from build123d import *

# Parameters (mm, degrees)
SURFACE_SKETCH_W         = 22.5
SURFACE_SKETCH_H         = 30
BODY_DEPTH               = 4.5
SKETCH_19_W              = 22.5
SKETCH_19_H              = 24
EXTRUDE_4_DEPTH          = 3
FILLET_6_R               = 1.5
MAGNET_CUTOUT_SKETCH_W   = 2.2
MAGNET_CUTOUT_SKETCH_H   = 6.2
MAGNET_CUTOUT_DEPTH      = 2.6
BORDER_DEPTH             = 0.5
CHAMPFER_DEPTH           = 22.5
FILLET_7_R               = 1.5
FILLET_8_R               = 0.5
CUT_EXTRUDE_1_DEPTH      = 23.5
CUT_EXTRUDE_2_DEPTH      = 1
CUT_EXTRUDE_2_DEPTH_BACK = 55


with BuildPart() as part:
    # surface_sketch → body (new body)
    with BuildSketch(Plane(origin=(0, 0, 0), x_dir=(1, 0, 0), z_dir=(0, 1, 0))):
        with Locations((-1.15, 0)):
            Rectangle(SURFACE_SKETCH_W, SURFACE_SKETCH_H)
    extrude(amount=-BODY_DEPTH)

    # Эскиз19 → Бобышка-Вытянуть4 (add)
    with BuildSketch(Plane(origin=(0, -4.5, 0), x_dir=(1, 0, 0), z_dir=(0, 1, 0))):
        with Locations((-1.15, -27)):
            Rectangle(SKETCH_19_W, SKETCH_19_H)
    extrude(amount=EXTRUDE_4_DEPTH)

    # Скругление6
    fillet_6_edges = [part.edges().sort_by_distance(p)[0] for p in [
        (-12.4, -3, 39),
        (10.1, -3, 39),
        (10.1, -2.25, -15),
        (-12.4, -2.25, -15),
    ]]
    fillet(fillet_6_edges, radius=FILLET_6_R)

    # magnet_cutout_sketch → magnet_cutout (cut)
    with BuildSketch(Plane.XZ.offset(4.5)):
        with Locations((9, 7.1)):
            Rectangle(MAGNET_CUTOUT_SKETCH_W, MAGNET_CUTOUT_SKETCH_H)
    magnet_cutout = extrude(amount=-MAGNET_CUTOUT_DEPTH, mode=Mode.SUBTRACT)

    # magnet_cutout_mirror: magnet_cutout across plane
    add(magnet_cutout.mirror(Plane(origin=(-1.15, 0, 0), x_dir=(0, 0, 1), z_dir=(1, 0, 0))), mode=Mode.SUBTRACT)

    # border_sketch → border (add)
    with BuildSketch(Plane(origin=(0, 0, 0), x_dir=(1, 0, 0), z_dir=(0, 1, 0))):
        with BuildLine():
            Line((-12.4, -15), (-12.4, 13.5))
            ThreePointArc((-12.4, 13.5), (-11.960660172, 14.560660172), (-10.9, 15))
            Line((-10.9, 15), (8.6, 15))
            ThreePointArc((8.6, 15), (9.660660172, 14.560660172), (10.1, 13.5))
            Line((10.1, 13.5), (10.1, -15))
            Line((10.1, -15), (9.1, -15))
            Line((9.1, -15), (9.1, 13.5))
            ThreePointArc((9.1, 13.5), (8.953553391, 13.853553391), (8.6, 14))
            Line((8.6, 14), (-10.9, 14))
            ThreePointArc((-10.9, 14), (-11.253553391, 13.853553391), (-11.4, 13.5))
            Line((-11.4, 13.5), (-11.4, -15))
            Line((-11.4, -15), (-12.4, -15))
        make_face()
    extrude(amount=BORDER_DEPTH)

    # Эскиз21 → champfer (add)
    with BuildSketch(Plane.ZY.offset(12.4)):
        Polygon((15, 0.5), (17, -1.5), (15, -1.5), (14, -1.5), (14, 0.5), align=None)
    extrude(amount=-CHAMPFER_DEPTH)

    # Скругление7
    fillet_7_edges = [part.edges().sort_by_distance(p)[0] for p in [
        (-12.4, -0.5, 16),
        (10.1, -0.5, 16),
    ]]
    fillet(fillet_7_edges, radius=FILLET_7_R)

    # Скругление8
    fillet_8_edges = [part.edges().sort_by_distance(p)[0] for p in [
        (9.1, 0.25, 14),
        (-11.4, 0.25, 14),
    ]]
    fillet(fillet_8_edges, radius=FILLET_8_R)

    # Эскиз22 → Вырез-Вытянуть1 (cut, through all)
    with BuildSketch(Plane.ZY.offset(12.4)):
        with BuildLine():
            Line((12.878679656, 0.5), (14.378679656, 0.5))
            ThreePointArc((14.378679656, 0.5), (14.952704805, 0.385819299), (15.439339828, 0.060660172))
            Line((15.439339828, 0.060660172), (17, -1.5))
            Line((17, -1.5), (17.923275361, -1.5))
            Line((17.923275361, -1.5), (15.181180077, 1.242095285))
            Line((15.181180077, 1.242095285), (12.878679656, 1.122407091))
            Line((12.878679656, 1.122407091), (12.878679656, 0.5))
        make_face()
    extrude(amount=-CUT_EXTRUDE_1_DEPTH, mode=Mode.SUBTRACT)

    # Эскиз23 → Вырез-Вытянуть2 (cut, two sides)
    with BuildSketch(Plane(origin=(0, 0, -15), x_dir=(-1, 0, 0), z_dir=(0, 0, -1))) as cut_extrude_2_sk:
        Polygon((1.15, -4.5), (-0.85, -4.5), (1.15, -2.5), (3.15, -4.5), align=None)
    extrude(amount=CUT_EXTRUDE_2_DEPTH, mode=Mode.SUBTRACT)
    extrude(cut_extrude_2_sk.sketch, amount=-CUT_EXTRUDE_2_DEPTH_BACK, mode=Mode.SUBTRACT)


solid = part.part
Can you work these out from the model? Positions are in its coordinate system, mm. A direction names the side the tool comes from. Give positions to 0.01 mm unless a question says otherwise; leave off trailing zeros. Loops run counter-clockwise (first coordinate to the right, second up) from the corner with the lowest first, then second, coordinate; pieces in that order, holes last. Notation, with made-up numbers: (20.5, -30) -> (35.5, -30) arc R28 ccw to (35.5, 2) -> close; hole circle Ø10 at (69, -13.5). An arc over 180 degrees is marked (long way). Use one line per item in the form item = value.
1) I need wall thicknesses on line 1 along Z through (x, y) = (0.75, 0.05); line 2 along X through (y, z) = (0.2, 11); line 3 along Z through (x, y) = (8.5, -3.15). Which ranges of each line are inside material? Lowest first, please.
Answers:
line_1 = -15 to -14, 14 to 15.45
line_2 = -12.4 to -11.4, 9.1 to 10.1
line_3 = -15 to 4, 10.2 to 39
2) Will these pins go through, and if not, where does the flat tip stop? pin 1 (2 mm diameter, centred on y = -3, z = 8.5, fed in from -X); pin 2 (1.1 mm diameter, centred on x = -11.5, z = 8.5, fed in from -Y); pin 3 (7 mm diameter, centred on x = -6, z = 27.5, fed in from +Y).
Answers:
pin_1 = -10.2
pin_2 = -1.9
pin_3 = -1.5
3) If we section it at B-B (z = 12): Please give me the cut outline in (x, y), plus the area to 4 significant figures.
Answers:
outline = (-12.4, -4.5) -> (-3.15, -4.5) -> (-1.15, -2.5) -> (0.85, -4.5) -> (10.1, -4.5) -> (10.1, 0.5) -> (9.1, 0.5) -> (9.1, 0) -> (-11.4, 0) -> (-11.4, 0.5) -> (-12.4, 0.5) -> close
area = 98.25 mm²
4) For faces 1 (the face through (-2.14, -3.49, 11.62)), 2 (the face through (-11, -3, 4)), 3 (the face through (-1, 0, 0)), 4 (the face through (7.9, -3, 7)), which set-ups out of +Z, -Z, +X, -X, +Y, -Y let a thin tool reach every point of the face, with its end or its side?
Answers:
face_1 = +Z, -Z, -Y
face_2 = -X, -Y
face_3 = +Y
face_4 = +X, -Y
5) If we section it at D-D (z = 33.5): Please give me the cut outline in (x, y), plus the area to 3 significant figures.
Answers:
outline = (-12.4, -4.5) -> (-3.15, -4.5) -> (-1.15, -2.5) -> (0.85, -4.5) -> (10.1, -4.5) -> (10.1, -1.5) -> (-12.4, -1.5) -> close
area = 63.5 mm²
6) If we section it at A-A (y = -3.05): Please give me the cut outline in (x, z), plus the area to 3 significant figures.
Answers:
outline = (-12.4, -13.5) arc R1.5 ccw to (-10.9, -15) -> (-1.7, -15) -> (-1.7, 39) -> (-10.9, 39) arc R1.5 ccw to (-12.4, 37.5) -> (-12.4, 10.2) -> (-10.2, 10.2) -> (-10.2, 4) -> (-12.4, 4) -> close; (-0.6, -15) -> (8.6, -15) arc R1.5 ccw to (10.1, -13.5) -> (10.1, 4) -> (7.9, 4) -> (7.9, 10.2) -> (10.1, 10.2) -> (10.1, 37.5) arc R1.5 ccw to (8.6, 39) -> (-0.6, 39) -> close
area = 1,130 mm²
7) If we section it at C-C (x = -2): Please give me the cut outline in (y, z).
Answers:
outline = (-3.35, -15) -> (0.5, -15) -> (0.5, -14) -> (0, -14) -> (0, 14) -> (0.5, 14) -> (0.5, 14.38) arc R1.5 ccw to (0.06, 15.44) -> (-1.5, 17) -> (-1.5, 39) -> (-3.35, 39) -> close
